```python
from build123d import *

# Parameters (mm, degrees)
F0_W     = 110
F0_H     = 50
F0_R     = 4.1
F0_R_2   = 4.05
F0_R_3   = 4
F0_R_4   = 3.95
F0_R_5   = 3.9
F0_R_6   = 6.1
F0_R_7   = 6.05
F0_R_8   = 6
F0_R_9   = 5.95
F0_R_10  = 5.9
F1_DEPTH = 15


with BuildPart() as f1:
    # F0 (on Front) → F1 (new body)
    with BuildSketch(Plane.XZ):
        Rectangle(F0_W, F0_H)
        with Locations((-40, -10)):
            Circle(F0_R, mode=Mode.SUBTRACT)
        with Locations((-20, -10)):
            Circle(F0_R_2, mode=Mode.SUBTRACT)
        with Locations((0, -10)):
            Circle(F0_R_3, mode=Mode.SUBTRACT)
        with Locations((20, -10)):
            Circle(F0_R_4, mode=Mode.SUBTRACT)
        with Locations((40, -10)):
            Circle(F0_R_5, mode=Mode.SUBTRACT)
        with Locations((-40, 10)):
            Circle(F0_R_6, mode=Mode.SUBTRACT)
        with Locations((-20, 10)):
            Circle(F0_R_7, mode=Mode.SUBTRACT)
        with Locations((0, 10)):
            Circle(F0_R_8, mode=Mode.SUBTRACT)
        with Locations((20, 10)):
            Circle(F0_R_9, mode=Mode.SUBTRACT)
        with Locations((40, 10)):
            Circle(F0_R_10, mode=Mode.SUBTRACT)
    extrude(amount=F1_DEPTH)


solid = f1.part
```
Here's how the part is built. I have some questions about the finished solid (model axes, mm). Round coordinates to 2 decimals unless told otherwise and drop trailing zeros. Order: outer loops, then holes, each group sorted by start corner. A loop starts at its lowest first (then second) coordinate and runs counter-clockwise, first axis right, second up. Notation, with made-up numbers: (36.5, 76.5) -> (47.5, 76.5) arc R20 ccw to (47.5, 110.5) -> close; hole circle Ø11 at (67.5, 46). An arc over 180 degrees is marked (long way). Use a Markdown table: item, result. Add a question column.
(1) Suppose I cut it at A-A, the plane x = 20. Please give me the cut outline in (y, z), and give its area (3 significant figures).
(2) Suppose I cut it at D-D, the plane x = 0. Please give me the cut outline in (y, z), and give its area (3 significant figures).
(3) Suppose I cut it at B-B, the plane z = -10. Please give me the cut outline in (x, y), and give its area (3 significant figures).
(4) I need wall thicknesses on line 1 along Z through (x, y) = (20, -8); line 2 along Z through (x, y) = (-37, -10.5); line 3 along X through (y, z) = (-9.5, 11.5). Which ranges of each line are inside material? Lowest first, please.
(5) If we mould it in two halves opening along X, with no side actions, what happens to faces 1 (the face through (23.65, -7.4, -11.51)), 2 (the face through (-1, -7, 25)), 3 (the face through (-55, -7, 0))? For each: released by +X, released by -X, zero draft, split by the parting line, or undercut.
(6) Suppose I cut it at C-C, the plane y = -2.5. Count the separate pieces of the cut face and the enclosed holes in it, and give its area (3 significant figures).
Verdict:
| question | item | result |
|---|---|---|
| 1 | outline | (-15, -25) -> (0, -25) -> (0, -13.95) -> (-15, -13.95) -> close; (-15, -6.05) -> (0, -6.05) -> (0, 4.05) -> (-15, 4.05) -> close; (-15, 15.95) -> (0, 15.95) -> (0, 25) -> (-15, 25) -> close |
| 1 | area | 453 mm2 |
| 2 | outline | (-15, -25) -> (0, -25) -> (0, -14) -> (-15, -14) -> close; (-15, -6) -> (0, -6) -> (0, 4) -> (-15, 4) -> close; (-15, 16) -> (0, 16) -> (0, 25) -> (-15, 25) -> close |
| 2 | area | 450 mm2 |
| 3 | outline | (-55, -15) -> (-44.1, -15) -> (-44.1, 0) -> (-55, 0) -> close; (-35.9, -15) -> (-24.05, -15) -> (-24.05, 0) -> (-35.9, 0) -> close; (-15.95, -15) -> (-4, -15) -> (-4, 0) -> (-15.95, 0) -> close; (4, -15) -> (16.05, -15) -> (16.05, 0) -> (4, 0) -> close; (23.95, -15) -> (36.1, -15) -> (36.1, 0) -> (23.95, 0) -> close; (43.9, -15) -> (55, -15) -> (55, 0) -> (43.9, 0) -> close |
| 3 | area | 1,050 mm2 |
| 4 | line 1 | -25 to -13.95, -6.05 to 4.05, 15.95 to 25 |
| 4 | line 2 | -25 to -12.79, -7.21 to 4.69, 15.31 to 25 |
| 4 | line 3 | -55 to -45.91, -34.09 to -25.86, -14.14 to -5.81, 5.81 to 14.24, 25.76 to 34.29, 45.71 to 55 |
| 5 | face 1 | undercut |
| 5 | face 2 | zero draft |
| 5 | face 3 | released by -X |
| 6 | separate pieces | 1 |
| 6 | enclosed holes | 10 |
| 6 | area | 4,680 mm2 |
